```python
from build123d import *

# Parameters (mm, degrees)
F1_DEPTH = 8
F2_R     = 1.5
F3_DEPTH = 12.5
F4_SIZE  = 1.99999
F5_R     = 3
F6_DEPTH = 4
F8_DEPTH = 2


# Not quite as in the source:
# - a fillet or chamfer is up to 0.001 mm smaller than in the source, because OpenCascade refuses the exact size


with BuildPart() as f1:
    # F0 (on Front) → F1 (new body)
    with BuildSketch(Plane.XZ):
        Polygon((5.1, 5.1), (5.1, -5.1), (-5.1, -5.1), (-5.1, 5.1), (-4.1, 5.1), (-1.1, 5.1), (-1.1, 8.1), (-1.1, 17.1), (-4.1, 17.1), (-4.1, 8.1), (-5.1, 8.1), (-8.1, 8.1), (-8.1, -8.1), (8.1, -8.1), (8.1, 8.1), (2.9, 8.1), (2.9, 17.1), (-0.1, 17.1), (-0.1, 8.1), (-0.1, 5.1), align=None)
    extrude(amount=F1_DEPTH)

    # F2 (on face) → F3 (cut, symmetric)
    with BuildSketch(Plane.YZ.offset(-1.1)):
        with Locations((-3, 11.6)):
            Circle(F2_R)
    extrude(amount=F3_DEPTH, both=True, mode=Mode.SUBTRACT)

    # F4 (size 2 in the source; OpenCascade refuses exactly that, so slightly less here)
    f4_edges = [f1.edges().sort_by_distance(p)[0] for p in [
        (2.9, -4, 8.1),
    ]]
    chamfer(f4_edges, length=F4_SIZE)

    # F5 (on face) → F6 (cut)
    with BuildSketch(Plane.YZ.offset(2.9)):
        with Locations((-3, 11.6)):
            Circle(F5_R)
    extrude(amount=F6_DEPTH, mode=Mode.SUBTRACT)

    # F7 (on face) → F8 (join)
    with BuildSketch(Plane.XZ.offset(8)):
        Polygon((-4.1, 12.1), (-8.1, 8.1), (-4.1, 8.1), align=None)
    extrude(amount=-F8_DEPTH)


solid = f1.part
```
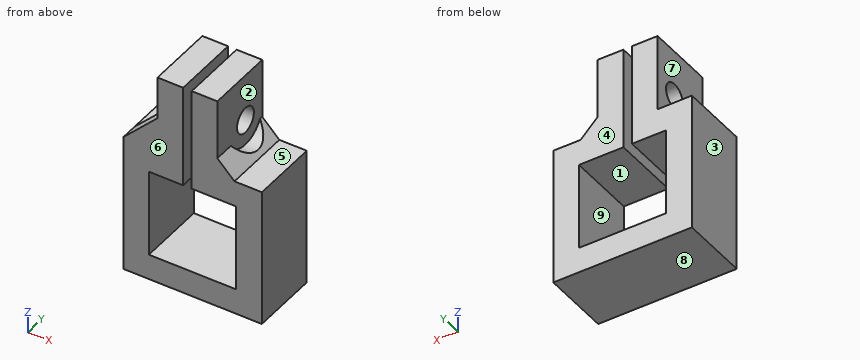
Check sheet for the modelled part. Datum: model origin and axes. Units: mm. Face numbers are marked on the shaded views. A direction names the side the tool comes from. Give positions to 0.01 mm unless a question says otherwise; leave off trailing zeros. Write each loop counter-clockwise with the first axis right and the second up, starting at its lowest first coordinate (ties: lowest second). Pieces come first, ordered by that corner, then holes. Notation, with made-up numbers: (31, 55.25) -> (86, 55.25) arc R12 ccw to (86, 74.25) -> close; hole circle Ø1 at (89.25, 10). An arc over 180 degrees is marked (long way). Use CSV: the item, a comma, the result in double quotes. Start each with the question number.
Q1. Cross-section at A-A on x = -2.5. Enter the section's corners in (y, z).
Q2. Release check for a two-part mould opening along X. For the marked faces 1, 2, 3 and 4 record: +X half, -X half, draft (parallel to the pull), parting line (faces both ways), or undercut.
Q3. Tool access check on the marked faces 5, 6, 7, 8 and 9. Record the directions out of +Z, -Z, +X, -X, +Y, -Y that give a thin tool (end or side, any length) a straight path to the whole face; none if there is none.
Q4. Scan lines: line 1 along Z through (x, y) = (1.2, -3); line 2 along X through (y, z) = (-6, 8); line 3 along X through (y, z) = (-5, 1.75). Record each from-to range of solid material in increasing order.
Q5. Depth check by flat-ended pin: P1, Ø1.8, axis at y = -3, z = 11.6, coming from the -X side; P2, Ø4, axis at y = -3.5, z = 14, coming from the +X side; P3, Ø2, axis at x = -6, y = -4.5, coming from the +Z side; P4, Ø2, axis at y = -4.5, z = 10.5, coming from the -X side. Enter the tip coordinate at first touch or a pass-through.
Q6. Cross-section at D-D on z = 11.6. Enter the section's corners in (x, y).
Q7. Cross-section at C-C on y = -3. Enter the section's corners in (x, z), and give its area (3 significant figures).
Q8. Cross-section at B-B on z = -1.75. Enter the section's corners in (x, y).
Working result:
1,outline,"(-8, -8.1) -> (0, -8.1) -> (0, -5.1) -> (-8, -5.1) -> close; (-8, 5.1) -> (0, 5.1) -> (0, 17.1) -> (-8, 17.1) -> close; hole circle Ø3 at (-3, 11.6)"
2,face 1,"undercut"
2,face 2,"+X half"
2,face 3,"-X half"
2,face 4,"draft"
3,face 5,"+Z, +X, +Y, -Y"
3,face 6,"+Z, -Z, +X, -X, -Y"
3,face 7,"+Z, -X, +Y"
3,face 8,"-Z, +X, -X, +Y, -Y"
3,face 9,"+Y, -Y"
4,line 1,"z = -8.1 to -5.1, 5.1 to 10.1, 13.1 to 17.1"
4,line 2,"x = -8.1 to -1.1, -0.1 to 8.1"
4,line 3,"x = -8.1 to -5.1, 5.1 to 8.1"
5,P1,"passes through"
5,P2,"stops at x = 2.9"
5,P3,"stops at z = 8.1"
5,P4,"stops at x = -4.1"
6,outline,"(-4.6, -8) -> (-1.1, -8) -> (-1.1, -4.5) -> (-4.1, -4.5) -> (-4.1, -6) -> (-4.6, -6) -> close; (-4.1, -1.5) -> (-1.1, -1.5) -> (-1.1, 0) -> (-4.1, 0) -> close; (-0.1, -8) -> (2.9, -8) -> (2.9, -4.5) -> (-0.1, -4.5) -> close; (-0.1, -1.5) -> (2.9, -1.5) -> (2.9, 0) -> (-0.1, 0) -> close"
7,outline,"(-8.1, -8.1) -> (8.1, -8.1) -> (8.1, 8.1) -> (4.9, 8.1) -> (4.4, 8.6) -> (2.9, 8.6) -> (2.9, 10.1) -> (-0.1, 10.1) -> (-0.1, 5.1) -> (5.1, 5.1) -> (5.1, -5.1) -> (-5.1, -5.1) -> (-5.1, 5.1) -> (-1.1, 5.1) -> (-1.1, 10.1) -> (-4.1, 10.1) -> (-4.1, 8.1) -> (-8.1, 8.1) -> close; (-4.1, 13.1) -> (-1.1, 13.1) -> (-1.1, 17.1) -> (-4.1, 17.1) -> close; (-0.1, 13.1) -> (2.9, 13.1) -> (2.9, 17.1) -> (-0.1, 17.1) -> close"
7,area,"192 mm^2"
8,outline,"(-8.1, -8) -> (-5.1, -8) -> (-5.1, 0) -> (-8.1, 0) -> close; (5.1, -8) -> (8.1, -8) -> (8.1, 0) -> (5.1, 0) -> close"
